Geometry: final body of the model. Coordinates: model frame, mm. A direction names the side the tool comes from. Coordinates: 2 decimals unless noted, no trailing zeros. Loops run counter-clockwise (first coordinate to the right, second up) from the corner with the lowest first, then second, coordinate; pieces in that order, holes last. Notation, with made-up numbers: (78.5, -28.5) - (95.5, -28.5) arc R9 cw to (95.5, -12.5) - close; hole circle Ø2 at (52, 57). An arc over 180 degrees is marked (long way). Put each result on its own line as item: value. Start each with the question number.
1) Draft query along Z for faces 1 (the flat face through (201, -9, 381)), 2 (the flat face through (-329.844, -9.392, 334.823)), 3 (the flat face through (65.85, -9.39, 468.66)), 4 (the flat face through (-5, 0, 335)). Return one class per face: +Z half, -Z half, draft (parallel to the pull), parting line (faces both ways), or undercut.
2) Material intervals for line 1 along Z through (x, y) = (125, -12.75); line 2 along X through (y, z) = (-9.5, 483); line 3 along X through (y, z) = (-3.5, 237), sorted ascending. Write a range as from..to.
3) Reachability of faces 5 (the flat face through (-129, -9, 101.6)), 6 (the flat face through (87.34, -9.39, 189.26)), 7 (the flat face through (-305, -9, 0)), 8 (the flat face through (-128, -9, 558.8)) from +Z, -Z, +X, -X, +Y, -Y: full face, straight path, thin tool, end or side. Return the list, or none.
4) Section C-C on x = -124.5. Output: boundary loops of the cut face in (y, z), and give its area (3 significant figures).
5) Section B-B on y = -9. Output: boundary loops of the cut face in (x, z).
6) Section A-A on x = 249. Output: boundary loops of the cut face in (y, z).
7) Section D-D on z = 289.5. Output: boundary loops of the cut face in (x, y), and give its area (3 significant figures).
8) Contact query for flat-ended pins moving along their axis: pin 1 Ø5.5 at (x, y) = (-80, -5.5) entering from -Z; pin 2 Ø8 at (y, z) = (-7, 237) entering from +X; pin 3 Ø1 at (y, z) = (-4, 141.5) entering from +X. Output: stop coordinate, or through.
```python
from build123d import *

# Parameters (mm, degrees)
F1_DEPTH = 19.05


with BuildPart() as f1:
    # F0 (on Front) → F1 (new body)
    with BuildSketch(Plane.XZ):
        Polygon((304.8, 660.4), (51.1001483644, 660.4), (58.9155329798, 558.8), (312.6153846154, 558.8), align=None)
        Polygon((94.084763749, 101.6), (101.9001483644, 0), (355.6, 0), (347.7846153846, 101.6), align=None)
        Polygon((-238.0690824048, 203.2), (-245.8844670202, 101.6), (-7.8153846154, 101.6), (-15.6307692308, 203.2), align=None)
        Polygon((326.2923076923, 381), (72.5924560567, 381), (80.4078406721, 279.4), (334.1076923077, 279.4), align=None)
        Polygon((-202.8998516356, 660.4), (-304.8, 660.4), (-355.6, 0), (-253.6998516356, 0), (-245.8844670202, 101.6), (-238.0690824048, 203.2), (-210.715236251, 558.8), align=None)
        Polygon((51.1001483644, 660.4), (-50.8, 660.4), (-42.9846153846, 558.8), (-15.6307692308, 203.2), (-7.8153846154, 101.6), (0, 0), (101.9001483644, 0), (94.084763749, 101.6), (80.4078406721, 279.4), (72.5924560567, 381), (58.9155329798, 558.8), align=None)
        Polygon((-50.8, 660.4), (-202.8998516356, 660.4), (-210.715236251, 558.8), (-42.9846153846, 558.8), align=None)
    extrude(amount=F1_DEPTH)


solid = f1.part
```
Answer block:
1. face 1: undercut
1. face 2: +Z half
1. face 3: undercut
1. face 4: draft
2. line 1: z = 0..101.6, 279.4..381, 558.8..660.4
2. line 2: x = -318.45..-216.55, -37.15..64.75
2. line 3: x = -337.37..-235.47, -18.23..83.67
3. face 5: -Z, +Y, -Y
3. face 6: +X, +Y, -Y
3. face 7: -Z, +X, -X, +Y, -Y
3. face 8: +Y, -Y
4. outline: (-19.05, 101.6) - (0, 101.6) - (0, 203.2) - (-19.05, 203.2) - close; (-19.05, 558.8) - (0, 558.8) - (0, 660.4) - (-19.05, 660.4) - close
4. area: 3,870 mm²
5. outline: (-355.6, 0) - (-253.7, 0) - (-245.88, 101.6) - (-7.82, 101.6) - (0, 0) - (355.6, 0) - (347.78, 101.6) - (94.08, 101.6) - (80.41, 279.4) - (334.11, 279.4) - (326.29, 381) - (72.59, 381) - (58.92, 558.8) - (312.62, 558.8) - (304.8, 660.4) - (-304.8, 660.4) - close; hole (-238.07, 203.2) - (-15.63, 203.2) - (-42.98, 558.8) - (-210.72, 558.8) - close
6. outline: (-19.05, 0) - (0, 0) - (0, 101.6) - (-19.05, 101.6) - close; (-19.05, 279.4) - (0, 279.4) - (0, 381) - (-19.05, 381) - close; (-19.05, 558.8) - (0, 558.8) - (0, 660.4) - (-19.05, 660.4) - close
7. outline: (-333.33, -19.05) - (-231.43, -19.05) - (-231.43, 0) - (-333.33, 0) - close; (-22.27, -19.05) - (333.33, -19.05) - (333.33, 0) - (-22.27, 0) - close
7. area: 8,720 mm²
8. pin 1: stops at z = 101.6
8. pin 2: stops at x = 83.98
8. pin 3: stops at x = 91.05
